Build history of the part. All positions in model axes, mm. Give positions to 0.01 mm unless a question says otherwise; leave off trailing zeros. Order: outer loops, then holes, each group sorted by start corner. A loop starts at its lowest first (then second) coordinate and runs counter-clockwise, first axis right, second up. Notation, with made-up numbers: M 84,24 L 107,24 A11 ccw 107,41 Z; hole C 82.25,-24.5 d3. An arc over 180 degrees is marked long. One line per item, written item: value.
from build123d import *

# Parameters (mm, degrees)
SKETCH1_R           = 25
SKETCH4_W           = 80.61138344
SKETCH4_H           = 104.08052039
BOSS_EXTRUDE1_DEPTH = 10


with BuildPart() as part:
    # Sweep1: sweep along a path in Sketch3
    with BuildLine(Plane(origin=(0, 0, 0), x_dir=(1, 0, 0), z_dir=(0, 1, 0))) as sweep1_path:
        Line((0, 0), (0, 500))
        ThreePointArc((0, 500), (29.289321881, 570.710678119), (100, 600))
        Line((100, 600), (1100, 600))
    # Sketch1 → Sweep1 (sweep)
    with BuildSketch(Plane.XY):
        Circle(SKETCH1_R)
    sweep(path=sweep1_path.line)

    # Sketch4 → Boss-Extrude1 (add)
    with BuildSketch(Plane(origin=(1100, 0, 0), x_dir=(0, 0, -1), z_dir=(1, 0, 0))):
        with Locations((602.803020109, -1.530595888)):
            Rectangle(SKETCH4_W, SKETCH4_H)
    extrude(amount=BOSS_EXTRUDE1_DEPTH)


solid = part.part
1) Saw through at A-A, the plane y = 0. Write the cut outline in (x, z), then the cut area to 3 significant figures.
Check values:
outline: M -25,-500 A125 ccw 100,-625 L 1100,-625 L 1100,-643.11 L 1110,-643.11 L 1110,-562.5 L 1100,-562.5 L 1100,-575 L 100,-575 A75 cw 25,-500 L 25,0 L -25,0 Z
area: 83,700 mm^2
2) Saw through at B-B, the plane x = 457. Write the cut outline in (y, z), then the cut area to 3 significant figures.
Check values:
outline: C 0,-600 d50
area: 1,960 mm^2
3) Saw through at C-C, the plane z = -435. Write the cut outline in (x, y), then the cut area to 3 significant figures.
Check values:
outline: C 0,0 d50
area: 1,960 mm^2
4) Mould opens along X. For faces 1 (the face through (23.846, -7.509, -253.5)), 2 (the face through (0, 0, 0)), 3 (the face through (1100, -24, -611)), 4 (the face through (607, -7.509, -576.154)) say: released by +X, released by -X, zero draft, split by the parting line, or undercut.
Check values:
face 1: split by the parting line
face 2: zero draft
face 3: undercut
face 4: undercut
5) Pin check, flat tips, straight feed: pin 1 (8 mm diameter, centred on x = 1102.5, y = -3, fed in from +Z); pin 2 (3 mm diameter, centred on x = 433.5, y = -10.5, fed in from -Z). Stop position of each tip, or through.
Check values:
pin 1: z = -562.5
pin 2: z = -623.32
6) Drill centre lines: probe 1 along Z at (x, y) = (501, -1.5); probe 2 along X at (y, z) = (29, -586); probe 3 along Z at (x, y) = (1058.5, -2). Where is each one in solid material? Low to high. Write a range as from..to.
Check values:
probe 1: -624.95..-575.05
probe 2: 1100..1110
probe 3: -624.92..-575.08
